from build123d import *

# Parameters (mm, degrees)
F0_R      = 457.2
F0_R_2    = 419.1
F1_DEPTH  = 1219.2
F5_R      = 10
F6_DEPTH  = 103
F7_R      = 7.5
F8_DEPTH  = 103
F9_R      = 2.5
F10_DEPTH = 101
F11_R     = 1
F12_DEPTH = 102
F13_R     = 2.5
F14_DEPTH = 103
F15_R     = 2.5
F16_DEPTH = 105
F17_R     = 5
F18_DEPTH = 103


with BuildPart() as f1:
    # F0 (on Front) → F1 (new body)
    with BuildSketch(Plane.XZ):
        Circle(F0_R)
        Circle(F0_R_2, mode=Mode.SUBTRACT)
    extrude(amount=F1_DEPTH)

    # F5 (on offset) → F6 (cut)
    with BuildSketch(Plane(origin=(319.1, 0, 0), x_dir=(0, -1, 0), z_dir=(-1, 0, 0))):
        with Locations((152.4, 0)):
            Circle(F5_R)
    extrude(amount=-F6_DEPTH, mode=Mode.SUBTRACT)

    # F7 (on offset) → F8 (cut)
    with BuildSketch(Plane(origin=(319.1, 0, 0), x_dir=(0, -1, 0), z_dir=(-1, 0, 0))):
        with Locations((304.8, 0)):
            Circle(F7_R)
    extrude(amount=-F8_DEPTH, mode=Mode.SUBTRACT)

    # F9 (on offset) → F10 (cut)
    with BuildSketch(Plane(origin=(319.1, 0, 0), x_dir=(0, -1, 0), z_dir=(-1, 0, 0))):
        with Locations((457.2, 0)):
            Circle(F9_R)
    extrude(amount=-F10_DEPTH, mode=Mode.SUBTRACT)

    # F11 (on offset) → F12 (cut)
    with BuildSketch(Plane(origin=(319.1, 0, 0), x_dir=(0, -1, 0), z_dir=(-1, 0, 0))):
        with Locations((609.6, 0)):
            Circle(F11_R)
    extrude(amount=-F12_DEPTH, mode=Mode.SUBTRACT)

    # F13 (on offset) → F14 (cut)
    with BuildSketch(Plane(origin=(319.1, 0, 0), x_dir=(0, -1, 0), z_dir=(-1, 0, 0))):
        with Locations((762, 0)):
            Circle(F13_R)
    extrude(amount=-F14_DEPTH, mode=Mode.SUBTRACT)

    # F15 (on offset) → F16 (cut)
    with BuildSketch(Plane(origin=(319.1, 0, 0), x_dir=(0, -1, 0), z_dir=(-1, 0, 0))):
        with Locations((914.4, 0)):
            Circle(F15_R)
    extrude(amount=-F16_DEPTH, mode=Mode.SUBTRACT)

    # F17 (on offset) → F18 (cut)
    with BuildSketch(Plane(origin=(319.1, 0, 0), x_dir=(0, -1, 0), z_dir=(-1, 0, 0))):
        with Locations((1066.8, 0)):
            Circle(F17_R)
    extrude(amount=-F18_DEPTH, mode=Mode.SUBTRACT)


solid = f1.part
Can you work these out from the model? Positions are in its coordinate system, mm. Give positions to 0.01 mm unless a question says otherwise; leave off trailing zeros. Write each loop counter-clockwise with the first axis right and the second up, starting at its lowest first coordinate (ties: lowest second). Pieces come first, ordered by that corner, then holes. Notation, with made-up numbers: (86, 60) -> (144, 60) arc R18 cw to (144, 67) -> close; hole circle Ø7 at (73, -24). An arc over 180 degrees is marked (long way). Answer as a JSON object with one key per item and string values. Group by question number.
Item 1: Please list where these lines run through material, in increasing order: line 1 (Y direction, x = 421.35, z = 0); line 2 (X direction, y = -310, z = 315); line 3 (X direction, y = -115, z = 165). Write a range as [from, to].
Item 2: Suppose I cut it at B-B (z = 89.5). Please give me the cut outline in (x, y), plus the area to 3 significant figures.
Item 3: I'm going to push flat-ended pins straight in: P1, Ø1.5, axis at x = 235, y = -1007, coming from the +Z side; P2, Ø1.5, axis at y = -281, z = 97, coming from the -X side; P3, Ø8, axis at x = 203.5, y = -880.5, coming from the -Z side. Where does each tip first touch, or does it pass through?
Item 4: Suppose I cut it at A-A (x = 0). Please give me the cut outline in (y, z), plus the area to 3 significant figures.
Item 5: Suppose I cut it at C-C (y = -532). Please give me the cut outline in (x, z), plus the area to 3 significant figures.
Item 6: We'd pull the mould along Z, two halves only. Please class faces 1 (the face through (201, -1219.2, -370)), 2 (the face through (-90.853, -601.066, -409.134)), 3 (the face through (-456.758, -601.066, 20.102)): +Z half, -Z half, draft (parallel to the pull), parting line (faces both ways), or undercut.
Findings:
{
 "1": {"line 1": "y = [-1219.2, -1071.8], [-1061.8, -916.9], [-911.9, -764.5], [-759.5, -312.3], [-297.3, -162.4], [-142.4, 0]", "line 2": "x = [-331.37, -276.44], [276.44, 331.37]", "line 3": "x = [-426.39, -385.25], [385.25, 426.39]"},
 "2": {"outline": "(-448.35, -1219.2) -> (-409.43, -1219.2) -> (-409.43, 0) -> (-448.35, 0) -> close; (409.43, -1219.2) -> (448.35, -1219.2) -> (448.35, 0) -> (409.43, 0) -> close", "area": "94,900 mm²"},
 "3": {"P1": "stops at z = 392.63", "P2": "stops at x = -446.95", "P3": "stops at z = -411.38"},
 "4": {"outline": "(-1219.2, -457.2) -> (0, -457.2) -> (0, -419.1) -> (-1219.2, -419.1) -> close; (-1219.2, 419.1) -> (0, 419.1) -> (0, 457.2) -> (-1219.2, 457.2) -> close", "area": "92,900 mm²"},
 "5": {"outline": "circle Ø914.4 at (0, 0); hole circle Ø838.2 at (0, 0)", "area": "105,000 mm²"},
 "6": {"face 1": "draft", "face 2": "undercut", "face 3": "parting line"}
}
